Solid Edge part; units mm, degrees
sketch "Sketch1" plane through (0, 0, 0) normal (0, 0, 1) x (1, 0, 0)
  circle A0 centre (0, 0) radius 15
extrude "Protrusion1" add sketch "Sketch1" along normal mid plane 180
hole "Bohrung_1" at (0, 0, -90) direction (0, 0, 1) diameter 10 depth 160
fillet "Round1" radius 1 4 edges at (-15, 0, 90) (-15, 0, -90) (0, -5, -90) (0, -5, 70)
properties material "Grafit"
Can you work these out from the model? Positions are in its coordinate system, mm. Give positions to 0.01 mm unless a question says otherwise; leave off trailing zeros. Loops run counter-clockwise (first coordinate to the right, second up) from the corner with the lowest first, then second, coordinate; pieces in that order, holes last. Notation, with made-up numbers: M -32.75,-0.75 L 7.25,-0.75 A21 ccw 7.25,7.25 Z; hole C -36,-38.75 d2. An arc over 180 degrees is marked long. Use CSV: the item, a comma, the result in double quotes. Start each with the question number.
1. If we mould it in two halves opening along X, with no side actions, what happens to faces 1 (the face through (-14.985, 0.66, 1.246)), 2 (the face through (4.88, -1.08, -8.89)), 3 (the face through (3, -6, -90)), 4 (the face through (0, 0, 70))? For each: released by +X, released by -X, zero draft, split by the parting line, or undercut.
2. For P1, Ø6.5, axis at x = 1, y = -1, coming from the -Z side; P2, Ø1.5, axis at x = 6.5, z = -10, coming from the -Y side; P3, Ø6, axis at x = -4, z = 6.5, coming from the +Y side, each with a flat end and sliding along its axis, tell me the tip position at first contact or that it passes through.
3. Imagine slicing it at A-A, the plane y = 0. Write out the boundary of the cut face in (x, z).
4. If I drill on L1, parallel to Y at x = 0, z = 6.5; L2, parallel to Y at x = 0, z = 80; L3, parallel to Y at x = -4, z = -38.5, over which ranges is the centre line in solid material (lowest first)?
5. Imagine slicing it at C-C, the plane z = 59. Write out the boundary of the cut face in (x, y).
Response values:
1,face 1,"split by the parting line"
1,face 2,"undercut"
1,face 3,"zero draft"
1,face 4,"undercut"
2,P1,"z = 69.75"
2,P2,"y = -13.85"
2,P3,"y = 14.97"
3,outline,"M -15,-89 A1 ccw -14,-90 L -6,-90 A1 ccw -5,-89 L -5,69 A1 cw -4,70 L 4,70 A1 cw 5,69 L 5,-89 A1 ccw 6,-90 L 14,-90 A1 ccw 15,-89 L 15,89 A1 ccw 14,90 L -14,90 A1 ccw -15,89 Z"
4,L1,"-15 to -5, 5 to 15"
4,L2,"-15 to 15"
4,L3,"-14.46 to -3, 3 to 14.46"
5,outline,"C 0,0 d30; hole C 0,0 d10"
